Autodesk Inventor part; units mm, degrees
ref_plane "YZ Plane" through (0, 0, 0) normal (1, 0, 0) x (0, 1, 0)
ref_plane "XZ Plane" through (0, 0, 0) normal (0, 1, 0) x (-1, 0, 0)
ref_plane "XY Plane" through (0, 0, 0) normal (0, 0, 1) x (1, 0, 0)
sketch "Sketch1" plane through (0, 0, 0) normal (0, 1, 0) x (-1, 0, 0)
  line L0 (7.8064, 7.8064) -> (173.9884, 7.8064) construction
  line L1 (173.9884, 7.8064) -> (173.9884, -141.9122) construction
  line L2 (173.9884, -141.9122) -> (7.8064, -141.9122) construction
  line L3 (7.8064, -141.9122) -> (7.8064, 7.8064) construction
  line L4 (7.5748, -142.1936) -> (54.8334, 7.8064)
  line L5 (54.8334, 7.8064) -> (72.4396, 7.8064)
  line L6 (72.4396, 7.8064) -> (122.7099, -142.1936)
  line L7 (122.7099, -142.1936) -> (104.0612, -142.1936)
  line L8 (104.0612, -142.1936) -> (89.8141, -96.7882)
  line L9 (89.8141, -96.7882) -> (38.1539, -96.7882)
  line L10 (38.1539, -96.7882) -> (24.8334, -142.1936)
  line L11 (24.8334, -142.1936) -> (7.5748, -142.1936)
  line L12 (42.9029, -80.572) -> (84.7176, -80.572)
  line L13 (84.7176, -80.572) -> (71.9763, -38.989)
  spline S0 degree 2 poles (71.9763, -38.989) (65.9531, -19.877) (63.289, -7.9465) knots 0 0 0 1 1 1
  spline S1 degree 2 poles (63.289, -7.9465) (60.8566, -22.4252) (56.5709, -36.5565) knots 0 0 0 1 1 1
  line L14 (56.5709, -36.5565) -> (42.9029, -80.572)
  point P0 (0, 0)
extrude "Extrusion1" add sketch "Sketch1" along normal blind 20
properties part number "Letter_A"
Input: part model. Units: mm. Frame: model coordinates. A direction names the side the tool comes from. Round coordinates to 2 decimals unless told otherwise and drop trailing zeros. Loops run counter-clockwise (first coordinate to the right, second up) from the corner with the lowest first, then second, coordinate; pieces in that order, holes last. Notation, with made-up numbers: M -13,-10.5 L 39,-10.5 A8 cw 39,-0.5 Z; hole C 32,40.5 d8. An arc over 180 degrees is marked long. Answer as CSV lines item,"result". Start each with the question number.
(1) First-contact query: pin 1 (2 mm diameter, centred on y = 7, z = -7.5, fed in from -X); pin 2 (4 mm diameter, centred on y = 9.5, z = -120.5, fed in from -X); pin 3 (1 mm diameter, centred on x = -42, y = 6.5, fed in from -Z). Flat tips, straight axial feed; report the tip coordinate or a pass-through.
(2) Line query: line 1 (X direction, y = 1.5, z = -97); line 2 (X direction, y = 3.25, z = -71.5); line 3 (X direction, y = 2.5, z = -3). Output: solid intervals per line, ascending. Write a range as [from, to].
(3) Section C-C, the plane x = -113. Output: boundary loops of the cut face in (y, z), plus the area to 3 significant figures.
(4) Reachability of faces 4 (the flat face through (-49.83, 9.86, -58.26)), 5 (the flat face through (-97.037, 9.86, -119.809)), 6 (the flat face through (-16, 10, -142.194)) from +Z, -Z, +X, -X, +Y, -Y: full face, straight path, thin tool, end or side. Return the list, or none.
(5) Section D-D, the plane x = -19. Output: boundary loops of the cut face in (y, z), plus the area to 3 significant figures.
(6) Section B-B, the plane z = -99. Output: boundary loops of the cut face in (x, y).
(7) Section A-A, the plane x = -49.5. Output: boundary loops of the cut face in (y, z).
(8) Draft query along Z for faces 1 (the flat face through (-31.587, 9.86, -119.173)), 2 (the flat face through (-30.873, 9.86, -68.244)), 3 (the flat face through (-78.436, 9.86, -60.072)). Return one class per face: released by +Z, released by -Z, zero draft, split by the parting line, or undercut.
Values found:
1,pin 1,"stops at x = -77.9"
1,pin 2,"stops at x = -116.11"
1,pin 3,"stops at z = -96.79"
2,line 1,"x = [-107.56, -89.88], [-38.09, -21.81]"
2,line 2,"x = [-99.02, -81.94], [-45.72, -29.85]"
2,line 3,"x = [-76.06, -51.43]"
3,outline,"M 0,-142.19 L 20,-142.19 L 20,-113.22 L 0,-113.22 Z"
3,area,"579 mm²"
4,face 4,"+Y, -Y"
4,face 5,"-Z, +Y, -Y"
4,face 6,"-Z, +X, -X, +Y, -Y"
5,outline,"M 0,-142.19 L 20,-142.19 L 20,-105.93 L 0,-105.93 Z"
5,area,"725 mm²"
6,outline,"M -108.23,0 L -90.51,0 L -90.51,20 L -108.23,20 Z; M -37.51,0 L -21.18,0 L -21.18,20 L -37.51,20 Z"
7,outline,"M 0,-96.79 L 20,-96.79 L 20,-80.57 L 0,-80.57 Z; M 0,-59.33 L 20,-59.33 L 20,-9.12 L 0,-9.12 Z"
8,face 1,"released by -Z"
8,face 2,"released by +Z"
8,face 3,"undercut"
